from build123d import *

# Parameters (mm, degrees)
BASE_FLANGE2_DEPTH = 300
SKETCH10_R         = 2.5
CUT_EXTRUDE1_DEPTH = 140


# Sheet-metal steps are written as plain solids
with BuildPart() as part:
    # Sketch1 → Base-Flange2 (new body)
    with BuildSketch(Plane.XY):
        with BuildLine():
            Line((-40, 76.091212948), (-48.5, 76.091212948))
            ThreePointArc((-48.5, 76.091212948), (-53.096194078, 74.187407026), (-55, 69.591212948))
            Line((-55, 69.591212948), (-55, 49.12471643))
            ThreePointArc((-55, 49.12471643), (-54.390131323, 46.375834295), (-52.67496831, 44.142785116))
            Line((-52.67496831, 44.142785116), (-4.17496831, 3.498715517))
            ThreePointArc((-4.17496831, 3.498715517), (0, 1.98064683), (4.17496831, 3.498715517))
            Line((4.17496831, 3.498715517), (52.67496831, 44.142785116))
            ThreePointArc((52.67496831, 44.142785116), (54.390131323, 46.375834295), (55, 49.12471643))
            Line((55, 49.12471643), (55, 69.591212948))
            ThreePointArc((55, 69.591212948), (53.096194078, 74.187407026), (48.5, 76.091212948))
            Line((48.5, 76.091212948), (40, 76.091212948))
            Line((40, 76.091212948), (40, 70.091212948))
            Line((40, 70.091212948), (48.5, 70.091212948))
            ThreePointArc((48.5, 70.091212948), (48.853553391, 69.944766339), (49, 69.591212948))
            Line((49, 69.591212948), (49, 49.12471643))
            ThreePointArc((49, 49.12471643), (48.953087025, 48.913263958), (48.821151408, 48.741490944))
            Line((48.821151408, 48.741490944), (0.321151408, 8.097421345))
            ThreePointArc((0.321151408, 8.097421345), (0, 7.98064683), (-0.321151408, 8.097421345))
            Line((-0.321151408, 8.097421345), (-48.821151408, 48.741490944))
            ThreePointArc((-48.821151408, 48.741490944), (-48.953087025, 48.913263958), (-49, 49.12471643))
            Line((-49, 49.12471643), (-49, 69.591212948))
            ThreePointArc((-49, 69.591212948), (-48.853553391, 69.944766339), (-48.5, 70.091212948))
            Line((-48.5, 70.091212948), (-40, 70.091212948))
            Line((-40, 70.091212948), (-40, 76.091212948))
        make_face()
    extrude(amount=-BASE_FLANGE2_DEPTH)

    # Sketch10 → Cut-Extrude1 (cut)
    with BuildSketch(Plane.ZY.offset(55)):
        with Locations(Location((-112.5, 59.12471643, 0), (0, 0, 180))):
            Circle(SKETCH10_R)
        with Locations(Location((-125, 59.12471643, 0), (0, 0, 180))):
            Circle(SKETCH10_R)
        with Locations(Location((-137.5, 59.12471643, 0), (0, 0, 180))):
            Circle(SKETCH10_R)
        with Locations(Location((-150, 59.12471643, 0), (0, 0, 180))):
            Circle(SKETCH10_R)
        with Locations(Location((-162.5, 59.12471643, 0), (0, 0, 180))):
            Circle(SKETCH10_R)
    extrude(amount=-CUT_EXTRUDE1_DEPTH, mode=Mode.SUBTRACT)


solid = part.part
Can you work these out from the model? Positions are in its coordinate system, mm. A direction names the side the tool comes from. Give positions to 0.01 mm unless a question says otherwise; leave off trailing zeros. Order: outer loops, then holes, each group sorted by start corner. A loop starts at its lowest first (then second) coordinate and runs counter-clockwise, first axis right, second up. Notation, with made-up numbers: M -39,16.25 L -2,16.25 A7 cw -2,20.25 Z; hole C -32.5,-20.5 d9. An arc over 180 degrees is marked long. Use one line per item in the form item = value. Start each with the question number.
Item 1: For faces 1 (the flat face through (-49, 61, -148)), 2 (the cylindrical face through (51.958, 58.374, -127.385)), 3 (the flat face through (40, 73, -148)), which set-ups out of +Z, -Z, +X, -X, +Y, -Y let a thin tool reach every point of the face, with its end or its side?
Item 2: We'd pull the mould along Z, two halves only. Please class faces 4 (the cylindrical face through (51.958, 58.374, -152.385)), 5 (the flat face through (-17, 20, 0)), 6 (the flat face through (-44, 70.091, -148)): +Z half, -Z half, draft (parallel to the pull), parting line (faces both ways), or undercut.
Item 3: If we section it at C-C (x = 10.5): Write out the boundary of the cut face in (y, z).
Item 4: If I drill on line 1 along X through (y, z) = (51, -116); line 2 along Y through (x, z) = (-53.45, -137.5); line 3 along Y through (x, z) = (-49.5, -112.5), over which ranges is the centre line in solid material (lowest first)?
Item 5: Will these pins go through, and if not, where does the flat tip stop? pin 1 Ø4 at (y, z) = (59.12, -112.5) entering from +X; pin 2 Ø3 at (x, z) = (8.5, -222.5) entering from -Y; pin 3 Ø3 at (y, z) = (73, -93) entering from +X; pin 4 Ø2.5 at (x, z) = (-45.5, -84.5) entering from -Y.
Item 6: If we section it at B-B (y = 39): Write out the boundary of the cut face in (x, z).
Item 7: If we section it at A-A (z = -156): Write out the boundary of the cut face in (x, y), then the cut area to 3 significant figures.
Outcome:
q1.face_1 = +Z, -Z
q1.face_2 = +X, -X
q1.face_3 = +Z, -Z, +Y
q2.face_4 = undercut
q2.face_5 = +Z half
q2.face_6 = draft
q3.outline = M 8.8,-300 L 16.63,-300 L 16.63,0 L 8.8,0 Z
q4.line_1 = -55 to -49, 49 to 55
q4.line_2 = 44.91 to 56.62, 61.62 to 73.8
q4.line_3 = 41.48 to 56.62, 61.62 to 76.01
q5.pin_1 = through
q5.pin_2 = 5.87
q5.pin_3 = 54.71
q5.pin_4 = 37.08
q6.outline = M -46.54,-300 L -37.2,-300 L -37.2,0 L -46.54,0 Z; M 37.2,-300 L 46.54,-300 L 46.54,0 L 37.2,0 Z
q7.outline = M -55,49.12 A6.5 ccw -52.67,44.14 L -4.17,3.5 A6.5 ccw 4.17,3.5 L 52.67,44.14 A6.5 ccw 55,49.12 L 55,69.59 A6.5 ccw 48.5,76.09 L 40,76.09 L 40,70.09 L 48.5,70.09 A0.5 cw 49,69.59 L 49,49.12 A0.5 cw 48.82,48.74 L 0.32,8.1 A0.5 cw -0.32,8.1 L -48.82,48.74 A0.5 cw -49,49.12 L -49,69.59 A0.5 cw -48.5,70.09 L -40,70.09 L -40,76.09 L -48.5,76.09 A6.5 ccw -55,69.59 Z
q7.area = 1,240 mm2
